```python
from build123d import *

# Parameters (mm, degrees)
F1_DEPTH = 44
F2_W     = 35.2
F2_H     = 20
F3_DEPTH = 20.001


with BuildPart() as f1:
    # F0 (on Front) → F1 (new body)
    with BuildSketch(Plane.XZ):
        with BuildLine():
            Line((-3, 0), (0, 0))
            Line((0, 0), (0, 119))
            ThreePointArc((0, 119), (0.8786796564, 121.1213203436), (3, 122))
            Line((3, 122), (17, 122))
            Line((17, 122), (17, 125))
            Line((17, 125), (3, 125))
            ThreePointArc((3, 125), (-1.2426406871, 123.2426406871), (-3, 119))
            Line((-3, 119), (-3, 0))
        make_face()
    extrude(amount=F1_DEPTH)

    # F2 (on face) → F3 (cut, through all)
    with BuildSketch(Plane(origin=(-3, 0, 0), x_dir=(0, -1, 0), z_dir=(-1, 0, 0))):
        with Locations((22, 129)):
            Rectangle(F2_W, F2_H)
    extrude(amount=-F3_DEPTH, mode=Mode.SUBTRACT)


solid = f1.part
```
Here's how the part is built. I have some questions about the finished solid (model axes, mm). A direction names the side the tool comes from. Coordinates: 2 decimals unless noted, no trailing zeros. Write each loop counter-clockwise with the first axis right and the second up, starting at its lowest first coordinate (ties: lowest second). Pieces come first, ordered by that corner, then holes. Notation, with made-up numbers: (-23, 2) -> (-1, 2) arc R31 cw to (-1, 29) -> close; hole circle Ø10 at (39, 84). An arc over 180 degrees is marked (long way). Use a Markdown table: item, result. Add a question column.
(1) Please list where these lines run through material, in increasing order: line 1 (X direction, y = -10, z = 57.5); line 2 (Z direction, x = -1.25, y = -21).
(2) We'd pull the mould along Y, two halves only. Please class faces 1 (the flat face through (7, -4.4, 123)), 2 (the flat face through (-0.5, -44, 72.1)), 3 (the flat face through (-3, -22, 60)): +Y half, -Y half, draft (parallel to the pull), parting line (faces both ways), or undercut.
(3) If we section it at C-C, the plane y = -10: Write out the boundary of the cut face in (x, z), and give its area (3 significant figures).
(4) If we section it at A-A, the plane x = 10.5: Write out the boundary of the cut face in (y, z), and give its area (3 significant figures).
(5) For faces 4 (the flat face through (7, -39.6, 123)), 5 (the flat face through (10, -2, 122)), 6 (the cylindrical face through (-1.196, -41.769, 123.289)), which set-ups out of +Z, -Z, +X, -X, +Y, -Y let a thin tool reach every point of the face, with its end or its side?
(6) I'm going to push flat-ended pins straight in: P1, Ø3, axis at y = -10, z = 109, coming from the +X side; P2, Ø0.9, axis at x = -1.5, y = -25.5, coming from the +Z side; P3, Ø2, axis at x = 13, y = -2, coming from the -Z side. Where does each tip first touch, or does it pass through?
(7) If we section it at B-B, the plane z = 95.5: Write out the boundary of the cut face in (x, y), and give its area (3 significant figures).
Outcome:
| question | item | result |
|---|---|---|
| 1 | line 1 | x = -3 to 0 |
| 1 | line 2 | z = 0 to 119 |
| 2 | face 1 | undercut |
| 2 | face 2 | -Y half |
| 2 | face 3 | draft |
| 3 | outline | (-3, 0) -> (0, 0) -> (0, 119) -> (-3, 119) -> close |
| 3 | area | 357 mm^2 |
| 4 | outline | (-44, 122) -> (-39.6, 122) -> (-39.6, 125) -> (-44, 125) -> close; (-4.4, 122) -> (0, 122) -> (0, 125) -> (-4.4, 125) -> close |
| 4 | area | 26.4 mm^2 |
| 5 | face 4 | +Z, +X, -X |
| 5 | face 5 | -Z, +X, +Y, -Y |
| 5 | face 6 | +Z, -X, +Y, -Y |
| 6 | P1 | stops at x = 0 |
| 6 | P2 | stops at z = 119 |
| 6 | P3 | stops at z = 122 |
| 7 | outline | (-3, -44) -> (0, -44) -> (0, 0) -> (-3, 0) -> close |
| 7 | area | 132 mm^2 |
